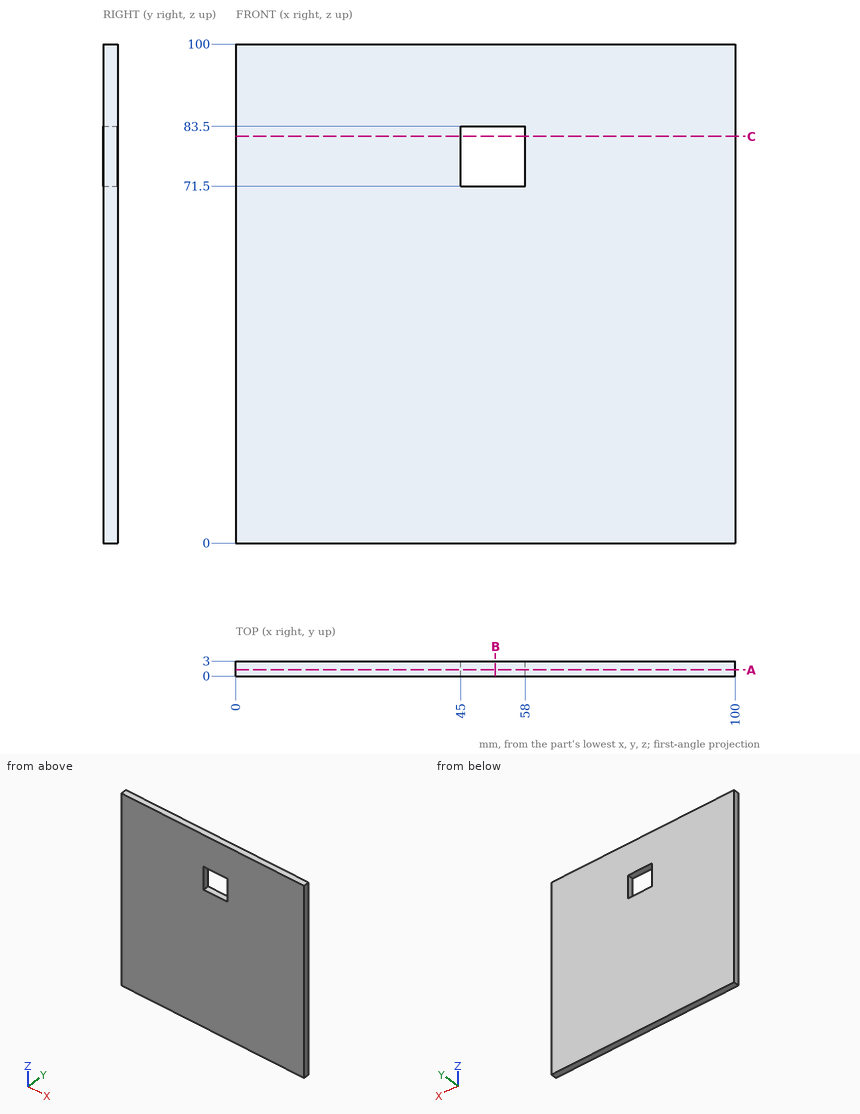
Design review of the part shown in the three views and the two pictorial views. Dimensions are in mm from the part's minimum x, y and z. Coordinates: 2 decimals unless noted, no trailing zeros. Write each loop counter-clockwise with the first axis right and the second up, starting at its lowest first coordinate (ties: lowest second). Pieces come first, ordered by that corner, then holes. Notation, with made-up numbers: (14.25, 36.5) -> (64.25, 36.5) arc R20 cw to (64.25, 59.5) -> close; hole circle Ø2 at (28.5, 58.25). An arc over 180 degrees is marked (long way). Answer in a Markdown table with one row per item.
1. We need section B-B, the plane x = 52. State the section outline as (y, z) points, and give its area (3 significant figures).
Answers below:
| item | result |
|---|---|
| outline | (0, 0) -> (3, 0) -> (3, 71.5) -> (0, 71.5) -> close; (0, 83.5) -> (3, 83.5) -> (3, 100) -> (0, 100) -> close |
| area | 264 mm^2 |
2. Wall thickness on probe 1 along Z at (x, y) = (50, 2.3); probe 2 along X at (y, z) = (2.3, 80.5): over which ranges is each line inside the solid? List them lowest first. Write a range as [from, to].
Answers below:
| item | result |
|---|---|
| probe 1 | z = [0, 71.5], [83.5, 100] |
| probe 2 | x = [0, 45], [58, 100] |
3. We need section A-A, the plane y = 1.25. State the section outline as (x, z) points.
Answers below:
| item | result |
|---|---|
| outline | (0, 0) -> (100, 0) -> (100, 100) -> (0, 100) -> close; hole (45, 71.5) -> (58, 71.5) -> (58, 83.5) -> (45, 83.5) -> close |
4. We need section C-C, the plane z = 81.5. State the section outline as (x, y) points, and give its area (3 significant figures).
Answers below:
| item | result |
|---|---|
| outline | (0, 0) -> (45, 0) -> (45, 3) -> (0, 3) -> close; (58, 0) -> (100, 0) -> (100, 3) -> (58, 3) -> close |
| area | 261 mm^2 |
